The listing builds one solid part. Answer for the finished solid, in the listing's coordinates (mm). A direction names the side the tool comes from. Coordinates: 2 decimals unless noted, no trailing zeros. Order: outer loops, then holes, each group sorted by start corner. A loop starts at its lowest first (then second) coordinate and runs counter-clockwise, first axis right, second up. Notation, with made-up numbers: (60.5, 59) - (100.5, 59) arc R17 ccw to (100.5, 78) - close; hole circle Ø6 at (29, 44). An arc over 180 degrees is marked (long way). Use a Markdown table: item, result. Add a question column.
Item 1: For faces 1 (the flat face through (34.807, 1, 0)), 2 (the cylindrical face through (-0.388, 1.513, 41.944)), 3 (the flat face through (-3, 6, 36)), determine the directions among +Z, -Z, +X, -X, +Y, -Y from which every point of the face is accessible in a straight line to the end or side of a thin tool.
Item 2: Find the intervals of material crossed by line 1 along Z through (x, y) = (35.5, 3); line 2 along X through (y, z) = (0.4, -17); line 3 along Z through (x, y) = (22, 4.7), in increasing order.
Item 3: The part is cut by section B-B, the plane x = 32.5. Give the vertices of the cut face in (y, z), then the cut area to 3 significant figures.
Item 4: The part is cut by section C-C, the plane y = 3. Give the vertices of the cut face in (x, z), then the cut area to 3 significant figures.
Item 5: Flat-ended cylindrical pins translate along their axes: P1, Ø1.8, axis at x = -4, y = 2.5, coming from the -Z side; P2, Ø1.8, axis at x = 7, y = 3.5, coming from the +Z side. Find the tip coordinate at first contact, or state that the pin passes through.
Item 6: The mould has two halves that part along X. Classify faces 4 (the flat face through (-35.193, 1, 0)), 5 (the cylindrical face through (-0.388, 1.513, -41.944)), 6 (the flat face through (0, 3, -46)): released by +X, released by -X, zero draft, split by the parting line, or undercut.
Item 7: The part is cut by section A-A, the plane z = -7.5. Give the vertices of the cut face in (x, y).
from build123d import *

# Parameters (mm, degrees)
SKETCH1_W               = 76
SKETCH1_H               = 76
SKETCH1_W_2             = 70
SKETCH1_H_2             = 70
EXTRUDE_THIN1_DEPTH     = 6
CUT_EXTRUDE1_DEPTH      = 83.516664984
CUT_EXTRUDE1_DEPTH_BACK = 83.516664984
SKETCH2_R               = 1.5
SKETCH3_R               = 1.5
BOSS_EXTRUDE1_DEPTH     = 8


with BuildPart() as part:
    # Sketch1 → Extrude-Thin1 (new body)
    with BuildSketch(Plane(origin=(0, 0, 0), x_dir=(1, 0, 0), z_dir=(0, 1, 0))):
        with Locations((-0.192988196, 0)):
            Rectangle(SKETCH1_W, SKETCH1_H)
        with Locations((-0.192988196, 0)):
            Rectangle(SKETCH1_W_2, SKETCH1_H_2, mode=Mode.SUBTRACT)
    extrude(amount=EXTRUDE_THIN1_DEPTH)

    # Sketch2 → Cut-Extrude1 (cut, two sides: drawn at the far end of the back side and taken through both)
    with BuildSketch(Plane.ZY.offset(-34.807011804).offset(-CUT_EXTRUDE1_DEPTH_BACK)):
        with Locations((0, 3)):
            Circle(SKETCH2_R)
    extrude(amount=CUT_EXTRUDE1_DEPTH + CUT_EXTRUDE1_DEPTH_BACK, mode=Mode.SUBTRACT)

    # Sketch3 → Boss-Extrude1 (add)
    with BuildSketch(Plane(origin=(0, 0, -38), x_dir=(-1, 0, 0), z_dir=(0, 0, -1))):
        with Locations(Location((0.192988196, 3, 0), (0, 0, 180))):
            Circle(SKETCH3_R)
    boss_extrude1 = extrude(amount=BOSS_EXTRUDE1_DEPTH)

    # Mirror1: Boss-Extrude1 across plane
    add(boss_extrude1.mirror(Plane.XY))


solid = part.part
Solution:
| question | item | result |
|---|---|---|
| 1 | face 1 | +Y, -Y |
| 1 | face 2 | +Z |
| 1 | face 3 | +Z, -Z, +X, -X, +Y |
| 2 | line 1 | z = -38 to -1.5, 1.5 to 38 |
| 2 | line 2 | x = -38.19 to -35.19, 34.81 to 37.81 |
| 2 | line 3 | z = -38 to -35, 35 to 38 |
| 3 | outline | (0, -38) - (6, -38) - (6, -35) - (0, -35) - close; (0, 35) - (6, 35) - (6, 38) - (0, 38) - close |
| 3 | area | 36.0 mm2 |
| 4 | outline | (-38.19, -38) - (-1.69, -38) - (-1.69, -46) - (1.31, -46) - (1.31, -38) - (37.81, -38) - (37.81, -1.5) - (34.81, -1.5) - (34.81, -35) - (-35.19, -35) - (-35.19, -1.5) - (-38.19, -1.5) - close; (-38.19, 1.5) - (-35.19, 1.5) - (-35.19, 35) - (34.81, 35) - (34.81, 1.5) - (37.81, 1.5) - (37.81, 38) - (1.31, 38) - (1.31, 46) - (-1.69, 46) - (-1.69, 38) - (-38.19, 38) - close |
| 4 | area | 906 mm2 |
| 5 | P1 | stops at z = -38 |
| 5 | P2 | stops at z = 38 |
| 6 | face 4 | undercut |
| 6 | face 5 | split by the parting line |
| 6 | face 6 | zero draft |
| 7 | outline | (-38.19, 0) - (-35.19, 0) - (-35.19, 6) - (-38.19, 6) - close; (34.81, 0) - (37.81, 0) - (37.81, 6) - (34.81, 6) - close |
